Geometry: final body of the model. Coordinates: model frame, mm. A direction names the side the tool comes from. Round coordinates to 2 decimals unless told otherwise and drop trailing zeros. Write each loop counter-clockwise with the first axis right and the second up, starting at its lowest first coordinate (ties: lowest second). Pieces come first, ordered by that corner, then holes. Notation, with made-up numbers: (39, 80.25) -> (65, 80.25) arc R35 ccw to (65, 113.25) -> close; hole circle Ø11 at (-14.75, -15). An arc over 180 degrees is marked (long way). One line per item, written item: value. Start each with the question number.
Autodesk Inventor part; units mm, degrees
ref_plane "YZ Plane" through (0, 0, 0) normal (1, 0, 0) x (0, 1, 0)
ref_plane "XZ Plane" through (0, 0, 0) normal (0, 1, 0) x (-1, 0, 0)
sketch "Sketch1" plane through (0, 0, 0) normal (0, 1, 0) x (-1, 0, 0)
  circle A0 centre (0, 0) radius 98.425
  circle A1 centre (0, 0) radius 102.489
  dimension "d0" = 196.85
  dimension "d1" = 4.064
extrude "Extrusion1" add sketch "Sketch1" along normal blind 8.255
sketch "Sketch2" plane through (0, 8.255, 0) normal (0, 1, 0) x (1, 0, 0)
  circle A0 centre (0, 0) radius 98.425
  circle A1 centre (0, 0) radius 98.425
  circle A2 centre (0, 0) radius 100.838
  dimension "d4" = 2.413
extrude "Extrusion2" add sketch "Sketch2" along normal blind 2.413
ref_plane "Work Plane1" through (0, 8.255, -100.838) normal (0, 0, 1) x (1, 0, 0)
sketch "Sketch3" plane through (0, 8.255, -100.838) normal (0, 0, 1) x (1, 0, 0)
  line L0 (102.489, 0) -> (-102.489, 0) construction
  line L1 (0, 0) -> (0, 1.27) construction
  point P0 (0, -8.255)
  dimension "d7" = 1.27
hole "Hole1" at (0, 9.525, -100.838) direction (0, 0, 1) diameter 1.5748 depth 6.2992 tip angle 118
pattern_circular "Circular Pattern1" count 6 over 360 about axis through (0, 0, 0) along (0, 1, 0) of "Hole1"
sketch "Sketch4" plane through (0, 0, 0) normal (0, -1, 0) x (1, 0, 0)
  circle A0 centre (0, 0) radius 100.33
  dimension "d18" = 200.66
extrude "Extrusion3" cut sketch "Sketch4" against normal blind 3.175
properties part number "4K sheild rim3" material "Brass, Soft Yellow"
(1) Line query: probe 1 along X at (y, z) = (3.25, 0.5); probe 2 along Z at (x, y) = (0, 2.15); probe 3 along Z at (x, y) = (0, 6) (3 decimals). Output: solid intervals per line, ascending.
(2) Section query A-A (z = -37.5). Output: boundary loops of the cut face in (x, y) (3 decimals), and give its area (3 significant figures).
(3) Pull-direction query (Z, two-part tool) for faces 4 (the face through (-100.74, 9.44, 4.43)), 5 (the face through (-68, 0, -75)), 6 (the face through (74, 3.175, -66)); classes: pulls with the +Z half, pulls with the -Z half, needs draft (parallel to the pull), parting line crosses it, or undercut.
(4) Set-up query: faces 1 (the face through (-75, 8.255, -68)), 2 (the face through (97, 10.668, 22)), 3 (the face through (-13.061, 1.565, 99.476)). Return all of +Z, -Z, +X, -X, +Y, -Y with unobstructed straight access to the full face (end or side cutting, diameter ignored); none if empty.
(5) Pin query (flat end, axial travel): pin 1 (6 mm diameter, centred on y = 4, z = 38.5, fed in from +X); pin 2 (1 mm diameter, centred on y = 9, z = -15, fed in from -X); pin 3 (4 mm diameter, centred on x = -33, y = 4, fed in from +Z); pin 4 (1.3 mm diameter, centred on x = 0, y = 9.525, fed in from +Z). Return the tip coordinate at first contact, or that it passes through.
(6) Section query C-C (z = -58). Output: boundary loops of the cut face in (x, y) (1 decimal), and give its area (3 significant figures).
Results list:
1. probe 1: x = -102.49 to -98.42, 98.42 to 102.49
1. probe 2: z = -102.49 to -100.33, 100.33 to 102.49
1. probe 3: z = -102.489 to -98.425, 98.425 to 102.489
2. outline: (-95.382, 0) -> (-93.058, 0) -> (-93.058, 3.175) -> (-91.001, 3.175) -> (-91.001, 10.668) -> (-93.606, 10.668) -> (-93.606, 8.255) -> (-95.382, 8.255) -> close; (91.001, 3.175) -> (93.058, 3.175) -> (93.058, 0) -> (95.382, 0) -> (95.382, 8.255) -> (93.606, 8.255) -> (93.606, 10.668) -> (91.001, 10.668) -> close
2. area: 71.8 mm^2
3. face 4: parting line crosses it
3. face 5: needs draft
3. face 6: undercut
4. face 1: +Y
4. face 2: +Z, -Z, +X, -X, +Y
4. face 3: -Y
5. pin 1: stops at x = 96.14
5. pin 2: stops at x = -99.79
5. pin 3: stops at z = 97.69
5. pin 4: passes through
6. outline: (-84.5, 0) -> (-81.9, 0) -> (-81.9, 3.2) -> (-79.5, 3.2) -> (-79.5, 10.7) -> (-82.5, 10.7) -> (-82.5, 8.3) -> (-84.5, 8.3) -> close; (79.5, 3.2) -> (81.9, 3.2) -> (81.9, 0) -> (84.5, 0) -> (84.5, 8.3) -> (82.5, 8.3) -> (82.5, 10.7) -> (79.5, 10.7) -> close
6. area: 81.6 mm^2
